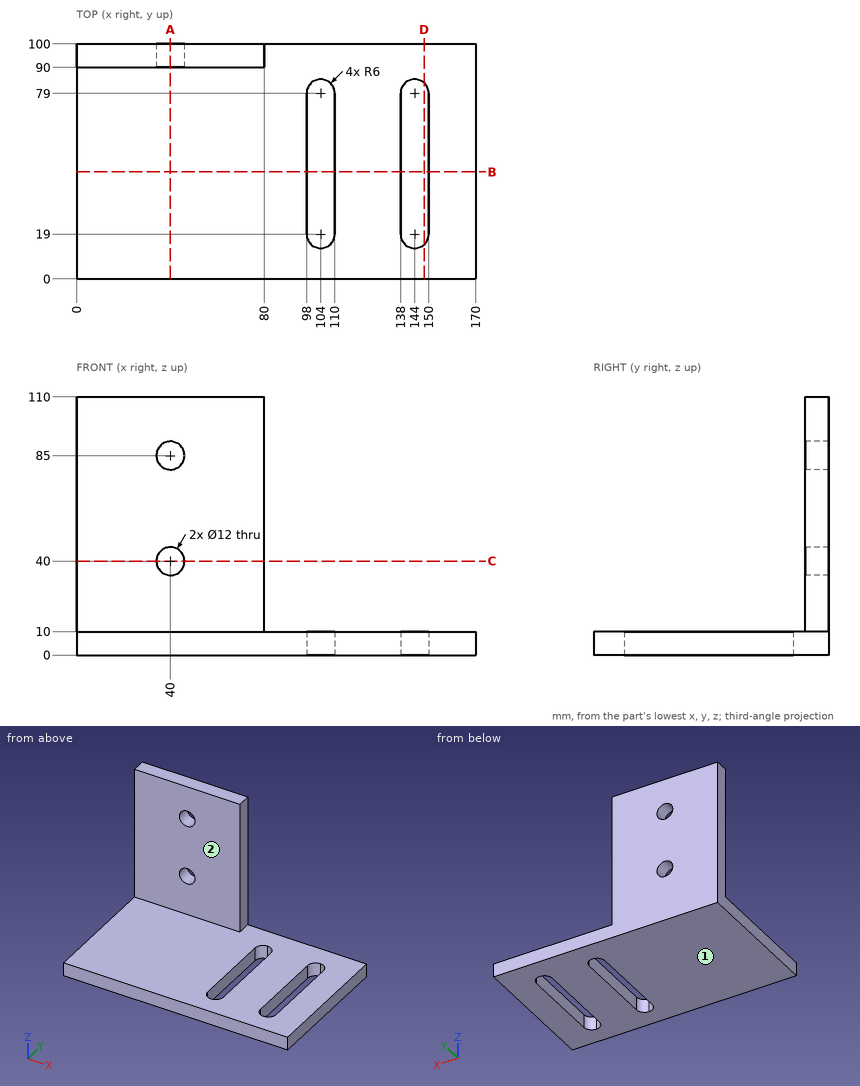
The drawing under review shows one solid part. Ordinate dimensions are in mm from its lowest x, y, z. A direction names the side the tool comes from. Coordinates: 2 decimals unless noted, no trailing zeros. Order: outer loops, then holes, each group sorted by start corner. A loop starts at its lowest first (then second) coordinate and runs counter-clockwise, first axis right, second up. Notation, with made-up numbers: (-39, -20.5) - (12, -20.5) arc R10 ccw to (12, -10.5) - close; hole circle Ø6 at (3, -16.5). An arc over 180 degrees is marked (long way). Put each result on its own line as item: value.
1) Take a section at A-A, the plane x = 40. Give the boundary of the cut face in (y, z).
Response values:
outline: (0, 0) - (100, 0) - (100, 34) - (90, 34) - (90, 10) - (0, 10) - close; (90, 46) - (100, 46) - (100, 79) - (90, 79) - close; (90, 91) - (100, 91) - (100, 110) - (90, 110) - close
2) Insertion check: P1, Ø8, axis at x = 144.5, y = 74, coming from the -Z side; P2, Ø14, axis at x = 40, z = 85, coming from the -Y side; P3, Ø2, axis at x = 90.5, y = 63, coming from the +Z side; P4, Ø3, axis at y = 95, z = 75.5, coming from the +X side. Each pin has a flat end and moves straight along its axis. Give the tip position at first contact, or say it passes through.
Response values:
P1: passes through
P2: stops at y = 90
P3: stops at z = 10
P4: stops at x = 80
3) Tool access review of the marked faces 1 and 2: name each direction out of +Z, -Z, +X, -X, +Y, -Y from which nothing blocks a thin tool from reaching the whole face with its end or side.
Response values:
face 1: -Z, +X, -X, +Y, -Y
face 2: +Z, +X, -X, -Y
4) Take a section at B-B, the plane y = 45.5. Give the boundary of the cut face in (x, z).
Response values:
outline: (0, 0) - (98, 0) - (98, 10) - (0, 10) - close; (110, 0) - (138, 0) - (138, 10) - (110, 10) - close; (150, 0) - (170, 0) - (170, 10) - (150, 10) - close
5) Wall thickness on L1, parallel to Z at x = 40, y = 93; L2, parallel to Y at x = 23, z = 58.5; L3, parallel to Z at x = 136.5, y = 45: over which ranges is each line inside the solid? List them lowest first. Write a range as from..to.
Response values:
L1: z = 0..34, 46..79, 91..110
L2: y = 90..100
L3: z = 0..10
6) Take a section at D-D, the plane x = 148. Give the boundary of the cut face in (y, z).
Response values:
outline: (0, 0) - (14.53, 0) - (14.53, 10) - (0, 10) - close; (83.47, 0) - (100, 0) - (100, 10) - (83.47, 10) - close
7) Take a section at C-C, the plane z = 40. Give the boundary of the cut face in (x, y).
Response values:
outline: (0, 90) - (34, 90) - (34, 100) - (0, 100) - close; (46, 90) - (80, 90) - (80, 100) - (46, 100) - close
